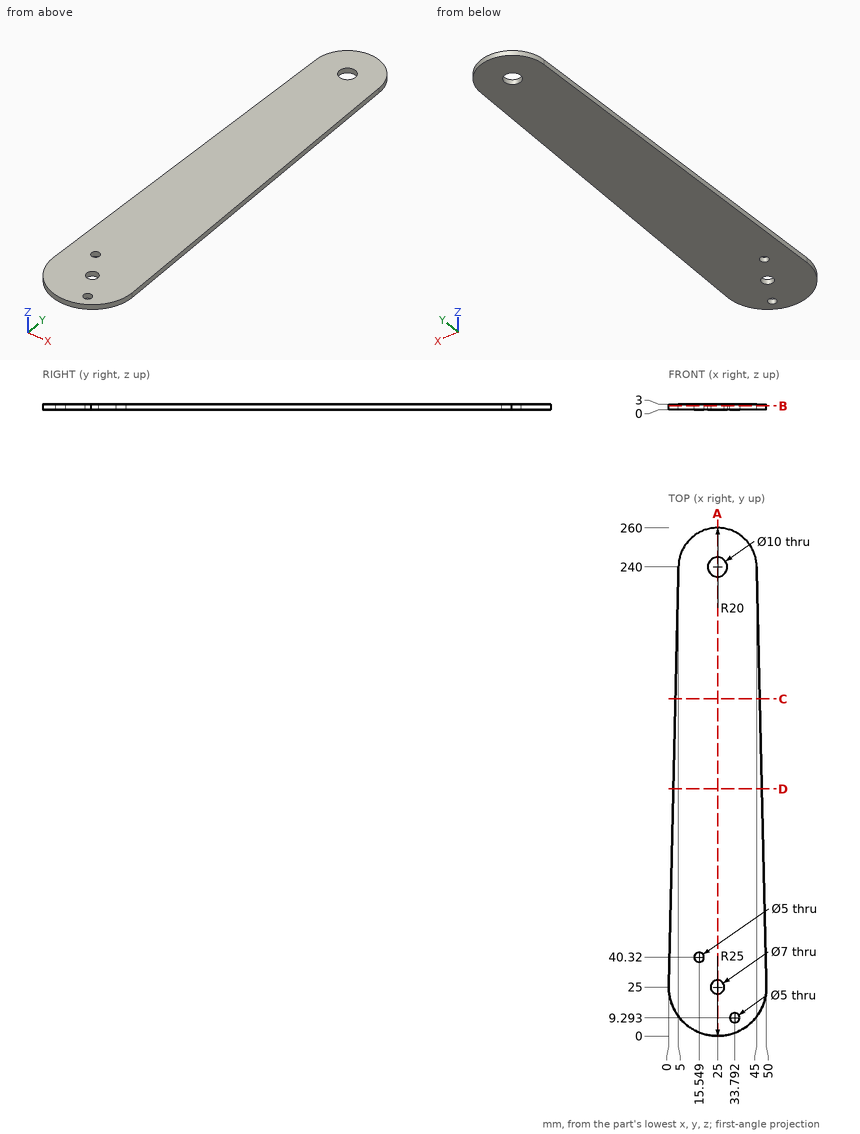
Verification items for this drawing (mm, ordinates from the low corner). Give positions to 0.01 mm unless a question says otherwise; leave off trailing zeros. Write each loop counter-clockwise with the first axis right and the second up, starting at its lowest first coordinate (ties: lowest second). Pieces come first, ordered by that corner, then holes. Notation, with made-up numbers: (-13.75, -28.5) -> (27.25, -28.5) arc R30 cw to (27.25, -5.5) -> close; hole circle Ø5 at (-18, 37.5). An arc over 180 degrees is marked (long way). Use one line per item in the form item = value.
Item 1: Sectioned sample at A-A on x = 25. Enter the section's corners in (y, z), plus the area to 3 significant figures.
Results list:
outline = (0, 0) -> (21.5, 0) -> (21.5, 3) -> (0, 3) -> close; (28.5, 0) -> (235, 0) -> (235, 3) -> (28.5, 3) -> close; (245, 0) -> (260, 0) -> (260, 3) -> (245, 3) -> close
area = 729 mm2
Item 2: Sectioned sample at D-D on y = 126.5. Enter the section's corners in (x, z), plus the area to 3 significant figures.
Results list:
outline = (2.36, 0) -> (47.64, 0) -> (47.64, 3) -> (2.36, 3) -> close
area = 136 mm2
Item 3: Sectioned sample at C-C on y = 172.5. Enter the section's corners in (x, z), plus the area to 3 significant figures.
Results list:
outline = (3.43, 0) -> (46.57, 0) -> (46.57, 3) -> (3.43, 3) -> close
area = 129 mm2
Item 4: Sectioned sample at B-B on z = 2.05. Enter the section's corners in (x, y), plus the area to 3 significant figures.
Results list:
outline = (0, 25) arc R25 ccw to (50, 25) -> (45, 240) arc R20 ccw to (5, 240) -> close; hole circle Ø5 at (15.55, 40.32); hole circle Ø10 at (25, 240); hole circle Ø7 at (25, 25); hole circle Ø5 at (33.79, 9.29)
area = 11,100 mm2
Item 5: Scan lines: line 1 (Y direction, x = 25, z = 1.75); line 2 (Y direction, x = 21, z = 2.75) (1 decimal); line 3 (Y direction, x = 26, z = 1.35) (1 decimal). Record each from-to range of solid material in increasing order.
Results list:
line_1 = 0 to 21.5, 28.5 to 235, 245 to 260
line_2 = 0.3 to 237, 243 to 259.6
line_3 = 0 to 21.6, 28.4 to 235.1, 244.9 to 260
Item 6: Depth check by flat-ended pin: pin 1 Ø1.5 at (x, z) = (45, 1) entering from -Y; pin 2 Ø5.5 at (x, y) = (25, 25) entering from -Z; pin 3 Ø1 at (x, z) = (10.5, 0.5) entering from -Y; pin 4 Ø6 at (x, y) = (15.55, 40.32) entering from -Z. Enter the tip coordinate at first touch or a pass-through.
Results list:
pin_1 = 9.05
pin_2 = through
pin_3 = 4.29
pin_4 = 0
